Design review of the part built by this model. Coordinates are the model's own, in mm. A direction names the side the tool comes from. Coordinates: 2 decimals unless noted, no trailing zeros. Write each loop counter-clockwise with the first axis right and the second up, starting at its lowest first coordinate (ties: lowest second). Pieces come first, ordered by that corner, then holes.
Q1. To check wall thickness, follow probe 1 along Y at (x, z) = (14.5, 3) (3 decimals); probe 2 along Y at (x, z) = (17.75, 52); probe 3 along X at (y, z) = (-20.5, -34). State the ranges of each line that lie inside material, in increasing order.
Q2. The part is to be moulded in two halves that separate along Y. For faces 4 (the face through (11, 22.225, -1)), 5 (the face through (2, -22.225, 96)), 6 (the face through (2, 22.225, 96)), say which applies: +Y half, -Y half, draft (parallel to the pull), parting line (faces both ways), or undercut.
Q3. Add section A-A, the plane x = 12.25. Give the boundary of the cut face in (y, z) (3 decimals), plus the area to 3 significant figures.
Q4. Clearance check with flat-ended pins moving along their axes: pin 1 Ø12.5 at (y, z) = (7, 13) entering from +X; pin 2 Ø2.5 at (x, y) = (10, -23) entering from +Z; pin 3 Ø2.5 at (x, y) = (13.5, 24) entering from -Z; pin 4 Ø1 at (y, z) = (-19, -9.5) entering from -X. State where each tip first meets the part, or that it passes through.
Q5. Add section C-C, the plane y = 11.5. Give the boundary of the cut face in (x, z).
Q6. Machinability: for faces 1 (the face through (11, -22.225, -1)), 2 (the face through (2, -22.225, -96)), 3 (the face through (2, 22.225, -96)), which of the approach directions +Z, -Z, +X, -X, +Y, -Y give a long, thin tool a straight path to every point of the face, cutting with its end or side? Answer none if there is none.
Autodesk Inventor part; units mm, degrees
ref_plane "YZ Plane" through (0, 0, 0) normal (1, 0, 0) x (0, 1, 0)
ref_plane "XZ Plane" through (0, 0, 0) normal (0, 1, 0) x (-1, 0, 0)
ref_plane "XY Plane" through (0, 0, 0) normal (0, 0, 1) x (1, 0, 0)
sketch "Sketch3" plane through (0, 0, 0) normal (0, 0, 1) x (1, 0, 0)
  line L0 (0, 25.4) -> (0, -25.4)
  line L1 (0, 25.4) -> (19.05, 25.4)
  line L2 (19.05, 25.4) -> (19.05, 22.225)
  line L3 (19.05, 22.225) -> (3.048, 22.225)
  line L4 (3.048, 22.225) -> (3.048, -22.225)
  line L5 (3.048, -22.225) -> (19.05, -22.225)
  line L6 (19.05, -22.225) -> (19.05, -25.4)
  line L7 (19.05, -25.4) -> (0, -25.4)
  line L8 (0, 0) -> (3.048, 0) construction
  dimension "d7" = 50.8
  dimension "d19" = 16.002
  dimension "d20" = 19.05
  dimension "d21" = 3.175
extrude "Extrusion3" add sketch "Sketch3" along normal mid plane 209.296
fillet "Fillet1" radius 1.5875 4 edges at (19.05, 22.225, 0) (19.05, -22.225, 0) (3.048, -22.225, 0) (3.048, 22.225, 0)
sketch "Sketch4" plane through (0, -25.4, 104.648) normal (-1, 0, 0) x (0, 0, 1)
  line L0 (0, 50.8) -> (-209.296, 50.8)
  line L1 (-209.296, 50.8) -> (-193.294, 50.8)
  line L2 (-193.294, 50.8) -> (-193.294, 47.625)
  line L3 (-193.294, 47.625) -> (-209.296, 47.625)
  line L4 (-209.296, 47.625) -> (-209.296, 50.8)
  line L5 (0, 46.0375) -> (-209.296, 46.0375)
  line L6 (-209.296, 4.7625) -> (0, 4.7625)
  line L7 (-209.296, 0) -> (0, 0)
  line L8 (-209.296, 0) -> (0, 0)
  line L9 (-209.296, 0) -> (-193.294, 0)
  line L10 (-193.294, 0) -> (-193.294, 3.175)
  line L11 (-193.294, 3.175) -> (-209.296, 3.175)
  line L12 (-209.296, 3.175) -> (-209.296, 0)
  line L13 (0, 3.175) -> (-209.296, 3.175)
  line L14 (-209.296, 47.625) -> (0, 47.625)
  point P0 (-104.648, 25.4)
  dimension "d14" = 16.002
extrude "Extrusion4" cut sketch "Sketch4" against normal through all
mirror "Mirror1" about plane through (0, 0, 0) normal (0, 0, 1) of "Extrusion4"
fillet "Fillet3" radius 1.5875 4 edges at (2.3177, 22.225, -104.648) (2.3177, -22.225, -104.648) (2.3177, 22.225, 104.648) (2.3177, -22.225, 104.648)
equation "\"d11\" = Length"
equation "\"Length\" = 209.296"
properties part number "NASA-20-FR-FP-01" material "Aluminum 6061"
Here are the results:
1. probe 1: y = -25.4 to -22.225, 22.225 to 25.4
1. probe 2: y = -25.4 to -22.25, 22.25 to 25.4
1. probe 3: x = 0 to 3.05
2. face 4: undercut
2. face 5: -Y half
2. face 6: +Y half
3. outline: (-25.4, -88.646) - (-22.225, -88.646) - (-22.225, 88.646) - (-25.4, 88.646) - close; (22.225, -88.646) - (25.4, -88.646) - (25.4, 88.646) - (22.225, 88.646) - close
3. area: 1,130 mm2
4. pin 1: stops at x = 3.05
4. pin 2: stops at z = 88.65
4. pin 3: stops at z = -88.65
4. pin 4: stops at x = 0
5. outline: (0, -104.65) - (3.05, -104.65) - (3.05, 104.65) - (0, 104.65) - close
6. face 1: +Z, -Z, +X
6. face 2: -Z, +X, -X, -Y
6. face 3: -Z, +X, -X, +Y
